For this review, take the finished solid that the model builds, in its own axes (mm). Face numbers are marked on the shaded views. A direction names the side the tool comes from. Give positions to 0.01 mm unless a question says otherwise; leave off trailing zeros. Loops run counter-clockwise (first coordinate to the right, second up) from the corner with the lowest first, then second, coordinate; pieces in that order, holes last. Notation, with made-up numbers: (61, -27.5) - (82, -27.5) arc R37 cw to (82, 11.5) - close; hole circle Ø8 at (-25.75, 46.25). An arc over 180 degrees is marked (long way). Use CSV: the item, a comma, the result in double quotes. Start each with the question number.
1. Take a section at A-A on y = 72. Give the boundary of the cut face in (x, z), plus the area to 4 significant figures.
2. Wall thickness on line 1 (Z direction, x = 34, y = 98.5); line 2 (X direction, y = 73, z = 64.5); line 3 (Y direction, x = 22.5, z = -8): over which ranges is each line inside the solid? List them lowest first.
3. Take a section at C-C on z = 136. Give the boundary of the cut face in (x, y), plus the area to 3 significant figures.
4. Mouldability with a two-part tool opening along Z and no side actions: class the marked faces 3, 4 and 5 as pulls with the +Z half, pulls with the -Z half, needs draft (parallel to the pull), parting line crosses it, or undercut.
5. Take a section at B-B on x = 27.5. Give the boundary of the cut face in (y, z), plus the area to 4 significant figures.
6. For pin 1 (12 mm diameter, centred on y = 48, z = 66, fed in from -X); pin 2 (10 mm diameter, centred on x = 35.5, z = 90.5, fed in from -Y); pin 3 (1 mm diameter, centred on y = 84, z = 93, fed in from -X), all flat-tipped, find the tip position at first contact; note any pin that passes through.
7. For the marked faces 1 and 2, list the 3-axis set-ups (+Z, -Z, +X, -X, +Y, -Y) from which the entire face can be reached by the end or side of a thin tool; tool diameter is ignored.
8. Take a section at D-D on y = 46. Give the boundary of the cut face in (x, z), plus the area to 3 significant figures.
Autodesk Inventor part; units mm, degrees
ref_plane "YZ Plane" through (0, 0, 0) normal (1, 0, 0) x (0, 1, 0)
ref_plane "XZ Plane" through (0, 0, 0) normal (0, 1, 0) x (-1, 0, 0)
ref_plane "XY Plane" through (0, 0, 0) normal (0, 0, 1) x (1, 0, 0)
sketch "草圖1" plane through (0, 0, 0) normal (0, 0, 1) x (1, 0, 0)
  circle A0 centre (0, 0) radius 95
  circle A1 centre (27.5, 72) radius 37.5
  dimension "d0" = 190
  dimension "d3" = 75
extrude "擠出1" add sketch "草圖1" along normal blind 160 contours A1 A0 | A0 A1 picked at (37.7638, 69.1742) picked at (30.5515, 96.5803)
sketch "草圖2" plane through (27.5, 72, 0) normal (0, 0, -1) x (-1, 0, 0)
  circle A0 centre (0, 0) radius 40
  point P0 (27.5, -72)
  dimension "d6" = 80
extrude "擠出2" add sketch "草圖2" against normal blind 10
sketch "草圖3" plane through (27.5, 72, 0) normal (0, 0, -1) x (-1, 0, 0)
  circle A0 centre (0, 0) radius 15
  point P0 (27.5, -72)
  dimension "d9" = 30
extrude "擠出3" add sketch "草圖3" along normal blind 80
properties part number "MotorPart2"
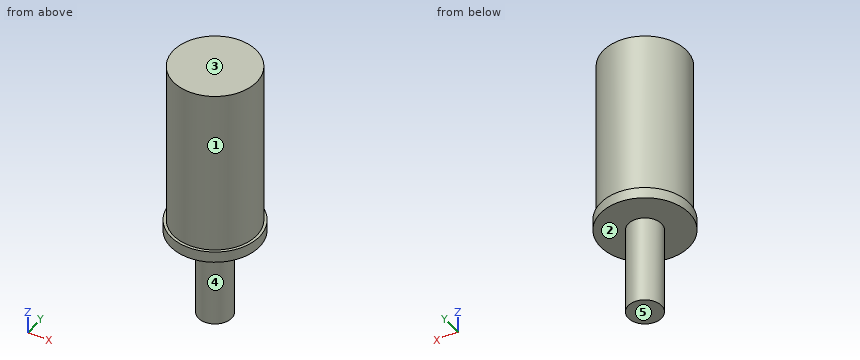
Check result:
1,outline,"(-12.5, 0) - (12.5, 0) - (12.5, -80) - (42.5, -80) - (42.5, 0) - (67.5, 0) - (67.5, 10) - (65, 10) - (65, 160) - (-10, 160) - (-10, 10) - (-12.5, 10) - close"
1,area,"14,450 mm²"
2,line 1,"z = 0 to 160"
2,line 2,"x = -9.99 to 64.99"
2,line 3,"y = 57.86 to 86.14"
3,outline,"circle Ø75 at (27.5, 72)"
3,area,"4,420 mm²"
4,face 3,"pulls with the +Z half"
4,face 4,"needs draft"
4,face 5,"pulls with the -Z half"
5,outline,"(32, 0) - (57, 0) - (57, -80) - (87, -80) - (87, 0) - (112, 0) - (112, 10) - (109.5, 10) - (109.5, 160) - (34.5, 160) - (34.5, 10) - (32, 10) - close"
5,area,"14,450 mm²"
6,pin 1,"stops at x = -5.4"
6,pin 2,"stops at y = 34.62"
6,pin 3,"stops at x = -8.19"
7,face 1,"+Z"
7,face 2,"-Z"
8,outline,"(-2.9, 0) - (57.9, 0) - (57.9, 10) - (54.52, 10) - (54.52, 160) - (0.48, 160) - (0.48, 10) - (-2.9, 10) - close"
8,area,"8,710 mm²"
